Part model, mm, in its own coordinate system. Face numbers are marked on the shaded views. A direction names the side the tool comes from. Round coordinates to 2 decimals unless told otherwise and drop trailing zeros. Order: outer loops, then holes, each group sorted by start corner. A loop starts at its lowest first (then second) coordinate and runs counter-clockwise, first axis right, second up. Notation, with made-up numbers: (13.5, -11) - (46.5, -11) arc R15 cw to (46.5, 6) - close; hole circle Ø11 at (32.5, 32). An arc over 180 degrees is marked (long way). Return JSON: item names as keys, results as strings. Group by question number.
Item 1: Drop flat-ended pins along their axis: pin 1 (5 mm diameter, centred on x = -13.5, y = -22, fed in from -Z); pin 2 (8 mm diameter, centred on x = -5, y = 22.5, fed in from -Z); pin 3 (8 mm diameter, centred on x = 14.5, y = 34.5, fed in from +Z); pin 4 (7 mm diameter, centred on y = 36.5, z = 0, fed in from +X). Give the stop position or say it passes through.
Item 2: Tool access for the marked faces 4, 5, 6 and 7: list every direction of +Z, -Z, +X, -X, +Y, -Y with a clear straight run to the whole face (end or side of a thin tool).
Item 3: Saw through at B-B on x = -23. List the corners of the cut face in (y, z).
Item 4: Probe probe 1 along Y at (x, z) = (-7, 0); probe 2 along Y at (x, z) = (8.5, 0); probe 3 along X at (y, z) = (54.5, 3.5). List the from-to ranges inside material, lowest first.
Item 5: Saw through at A-A on x = -12. List the corners of the cut face in (y, z), and give its area (3 significant figures).
Item 6: Two-plate mould, pull along Z, no slides. Class the marked faces 1, 2 and 3: released by +Z, released by -Z, zero draft, split by the parting line, or undercut.
```python
from build123d import *
from build123d.topology import SkipClean

# Parameters (mm, degrees)
EXTRUDE_1_DEPTH         = 10
EXTRUDE_1_DEPTH_BACK    = 17
SKETCH_1_R              = 61
SKETCH_3_R              = 25
EXTRUDE_2_DEPTH         = 19
SKETCH_4_R              = 21
EXTRUDE_3_DEPTH         = 6
SKETCH_5_R              = 16.2
CUT_EXTRUDE_1_DEPTH     = 11
SKETCH_6_R              = 14
CUT_EXTRUDE_2_DEPTH     = 96.514396821
HOLE_WIZARD_M10_1_D     = 8.5
HOLE_WIZARD_M10_1_DEPTH = 17.446342369
HOLE_WIZARD_M10_1_TIP   = 2.553657631
SKETCH_10_R             = 42.19592905
UNDEF_DEPTH             = 3
SKETCH_11_R             = 34
EXTRUDE_5_DEPTH         = 19
CUT_EXTRUDE_3_DEPTH     = 114.657379875
CHAMFER_1_SIZE          = 1


with BuildPart() as part:
    # Sketch 1 → Extrude 1 (new, two sides: drawn at the far end of the back side and taken through both)
    with BuildSketch(Plane(origin=(0, 0, 0), x_dir=(0, 0, -1), z_dir=(1, 0, 0)).offset(-EXTRUDE_1_DEPTH_BACK)):
        Circle(SKETCH_1_R)
    extrude(amount=EXTRUDE_1_DEPTH + EXTRUDE_1_DEPTH_BACK)

    # Sketch 2 → Cut-Revolve 1 (revolve, cut)
    with BuildSketch(Plane(origin=(0, 0, 0), x_dir=(1, 0, 0), z_dir=(0, 1, 0)), mode=Mode.PRIVATE) as cut_revolve_1_sk:
        Polygon((-6.570057385, 61), (-2.748423867, 48.5), (2.748423867, 48.5), (6.570057385, 61), align=None)
    revolve(cut_revolve_1_sk.sketch.rotate(Axis((0, 0, 0), (1, 0, 0)), 180), axis=Axis((0, 0, 0), (1, 0, 0)), mode=Mode.SUBTRACT)

    # Sketch 3 → Extrude 2 (add)
    with BuildSketch(Plane.ZY.offset(17)):
        Circle(SKETCH_3_R)
    extrude(amount=EXTRUDE_2_DEPTH)

    # Sketch 4 → Extrude 3 (add)
    with BuildSketch(Plane.ZY.offset(36)):
        Circle(SKETCH_4_R)
    extrude(amount=EXTRUDE_3_DEPTH)

    # Sketch 5 → Cut-Extrude 1 (cut)
    with BuildSketch(Plane.ZY.offset(42)):
        Circle(SKETCH_5_R)
    extrude(amount=-CUT_EXTRUDE_1_DEPTH, mode=Mode.SUBTRACT)

    # Sketch 6 → Cut-Extrude 2 (cut, through all)
    with BuildSketch(Plane.ZY.offset(31)):
        Circle(SKETCH_6_R)
    extrude(amount=-CUT_EXTRUDE_2_DEPTH, mode=Mode.SUBTRACT)

    # Hole Wizard M10 _1
    with Locations(Plane.ZY.offset(17)):
        with Locations((0, -36.5), (0, 36.5)):
            Hole(HOLE_WIZARD_M10_1_D / 2, depth=HOLE_WIZARD_M10_1_DEPTH)
            with Locations((0, 0, -(HOLE_WIZARD_M10_1_DEPTH + HOLE_WIZARD_M10_1_TIP / 2))):  # 118° drill point
                Cone(0, HOLE_WIZARD_M10_1_D / 2, HOLE_WIZARD_M10_1_TIP, mode=Mode.SUBTRACT)

    # Sketch 10 → undef (add)
    with BuildSketch(Plane(origin=(10, 0, 0), x_dir=(0, 0, -1), z_dir=(1, 0, 0))):
        Circle(SKETCH_10_R)
    extrude(amount=UNDEF_DEPTH)

    # Sketch 11 → Extrude 5 (add)
    with BuildSketch(Plane(origin=(13, 0, 0), x_dir=(0, 0, -1), z_dir=(1, 0, 0))):
        Circle(SKETCH_11_R)
    extrude(amount=EXTRUDE_5_DEPTH)

    # Sketch 12 → Cut-Revolve 2 (revolve, cut)
    with BuildSketch(Plane.XY, mode=Mode.PRIVATE) as cut_revolve_2_sk:
        Polygon((21.251576133, 21.5), (26.748423867, 21.5), (30.570057385, 34), (17.429942615, 34), align=None)
    revolve(cut_revolve_2_sk.sketch.rotate(Axis((0, 0, 0), (1, 0, 0)), 90), axis=Axis((0, 0, 0), (1, 0, 0)), mode=Mode.SUBTRACT)

    # Sketch 7 → Cut-Extrude 3 (cut, through all)
    with SkipClean():  # the faces are left unmerged after this step: merging them gives an invalid solid
        with BuildSketch(Plane.ZY.offset(42)):
            with BuildLine():
                Line((-4, 17.3), (4, 17.3))
                Line((4, 17.3), (4, 13.416407865))
                ThreePointArc((4, 13.416407865), (0, -14), (-4, 13.416407865))
                Line((-4, 13.416407865), (-4, 17.3))
            make_face()
        extrude(amount=-CUT_EXTRUDE_3_DEPTH, mode=Mode.SUBTRACT)
    add(part.part.scale(1), mode=Mode.REPLACE)  # the faces are merged on a copy

    # Chamfer 1
    chamfer_1_edges = [part.edges().sort_by_distance(p)[0] for p in [
        (-17, 0, 61),
        (32, -14, 0),
    ]]
    chamfer(chamfer_1_edges, length=CHAMFER_1_SIZE)


solid = part.part
```
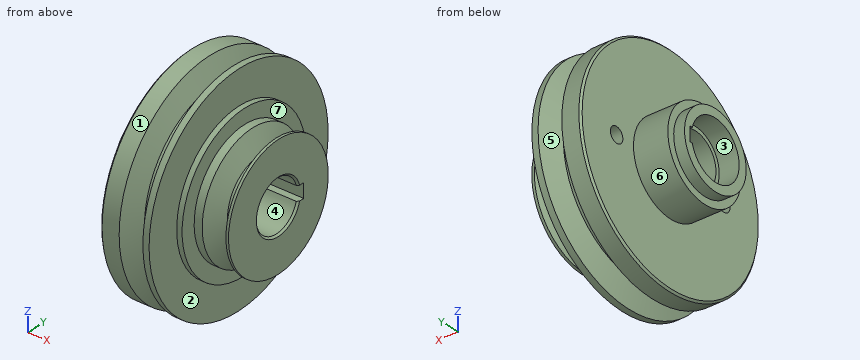
Filled in:
{
 "1": {"pin 1": "stops at z = -57.8", "pin 2": "stops at z = -58.02", "pin 3": "stops at z = 28.85", "pin 4": "stops at x = 32"},
 "2": {"face 4": "+X, -X", "face 5": "none", "face 6": "-X", "face 7": "+X"},
 "3": {"outline": "circle Ø50 at (0, 0); hole (13.42, -4) - (17.3, -4) - (17.3, 4) - (13.42, 4) arc R14 ccw (long way) to start"},
 "4": {"probe 1": "y = -61 to -40.75, -32.25 to -14, 17.3 to 32.25, 40.75 to 61", "probe 2": "y = -61 to -14, 17.3 to 61", "probe 3": "x = -17 to -4.62, 4.62 to 10"},
 "5": {"outline": "circle Ø122 at (0, 0); hole circle Ø8.5 at (-36.5, 0); hole (13.42, -4) - (17.3, -4) - (17.3, 4) - (13.42, 4) arc R14 ccw (long way) to start; hole circle Ø8.5 at (36.5, 0)", "area": "10,900 mm^2"},
 "6": {"face 1": "split by the parting line", "face 2": "zero draft", "face 3": "undercut"}
}
